```python
from build123d import *

# Parameters (mm, degrees)
F0_W     = 65
F0_H     = 12
F4_R     = 4.5
F5_DEPTH = 12


with BuildPart() as f1:
    # F0 (on Front) → F1 (revolve)
    with BuildSketch(Plane.XZ):
        with Locations((32.5, 6)):
            Rectangle(F0_W, F0_H)
    revolve(axis=Axis((0, 0, 18.457142), (0, 0, 1)))

    # F2 (on Front) → F3 (revolve, cut)
    with BuildSketch(Plane.XZ):
        Polygon((0, 12), (0, 0), (35, 0), (35, 6), (11, 6), (11, 8), (12.7, 8), (12.7, 12), align=None)
    revolve(axis=Axis((0, 0, 11.269168), (0, 0, 1)), mode=Mode.SUBTRACT)

    # F4 (on face) → F5 (cut, through all)
    with BuildSketch(Plane.XY.offset(12)):
        with Locations((55, 0)):
            Circle(F4_R)
        with Locations((0, 55)):
            Circle(F4_R)
        with Locations((-55, 0)):
            Circle(F4_R)
        with Locations((0, -55)):
            Circle(F4_R)
    extrude(amount=-F5_DEPTH, mode=Mode.SUBTRACT)


solid = f1.part
```
Verification items for the finished model (mm, model axes). A direction names the side the tool comes from. Coordinates: 2 decimals unless noted, no trailing zeros. Write each loop counter-clockwise with the first axis right and the second up, starting at its lowest first coordinate (ties: lowest second). Pieces come first, ordered by that corner, then holes. Notation, with made-up numbers: (-3.5, -33.5) - (53.5, -33.5) arc R7 cw to (53.5, -21.5) - close; hole circle Ø9 at (-14.75, 44). An arc over 180 degrees is marked (long way). One line per question, with ' | ' between items. Start each with the question number.
1. Section check A-A (y = 0). Enter the section's corners in (x, z).
2. Material ranges on line 1 along Y through (x, z) = (0, 7.05); line 2 along Y through (x, z) = (0, 4); line 3 along Y through (x, z) = (31.5, 1.5), recorded low to high.
3. Section check D-D (x = 52). Enter the section's corners in (y, z), plus the area to 4 significant figures.
4. Access from +Z, -Z, +X, -X, +Y, -Y to the whole of each face (thin tool, end or side, straight path). Record for faces 4 (the cylindrical face through (-2.75, -12.4, 10.03)), 5 (the cylindrical face through (-2.38, -10.74, 7.01)), 6 (the flat face through (-8, 8, 6)).
5. Draft check along X on faces 1 (the flat face through (0.1, 11.3, 8)), 2 (the cylindrical face through (62, 19.52, 6.08)), 3 (the flat face through (-28, -28, 0)). Enter one of: released by +X, released by -X, zero draft, split by the parting line, or undercut.
6. Gauge pin test, flat ends, axial feed: P1, Ø12, axis at x = -0.5, y = 18.5, coming from the -Z side; P2, Ø11.5, axis at x = 0, y = -55, coming from the +Z side; P3, Ø1, axis at x = 41, z = 5, coming from the +Y side; P4, Ø6, axis at x = -32, z = 10.5, coming from the -Y side. Record the tip position at first contact, or that the pin passes through.
7. Section check C-C (z = 3). Enter the section's corners in (x, y).
Computed values:
1) outline: (-65, 0) - (-59.5, 0) - (-59.5, 12) - (-65, 12) - close; (-50.5, 0) - (-35, 0) - (-35, 6) - (-11, 6) - (-11, 8) - (-12.7, 8) - (-12.7, 12) - (-50.5, 12) - close; (11, 6) - (35, 6) - (35, 0) - (50.5, 0) - (50.5, 12) - (12.7, 12) - (12.7, 8) - (11, 8) - close; (59.5, 0) - (65, 0) - (65, 12) - (59.5, 12) - close
2) line 1: -65 to -59.5, -50.5 to -11, 11 to 50.5, 59.5 to 65 | line 2: -65 to -59.5, -50.5 to -35, 35 to 50.5, 59.5 to 65 | line 3: -56.86 to -15.26, 15.26 to 56.86
3) outline: (-39, 0) - (-3.35, 0) - (-3.35, 12) - (-39, 12) - close; (3.35, 0) - (39, 0) - (39, 12) - (3.35, 12) - close | area: 855.5 mm²
4) face 4: +Z | face 5: +Z, -Z | face 6: -Z
5) face 1: undercut | face 2: split by the parting line | face 3: zero draft
6) P1: z = 6 | P2: z = 12 | P3: y = 50.84 | P4: y = -58.17
7) outline: circle Ø130 at (0, 0); hole circle Ø9 at (-55, 0); hole circle Ø70 at (0, 0); hole circle Ø9 at (0, -55); hole circle Ø9 at (0, 55); hole circle Ø9 at (55, 0)
